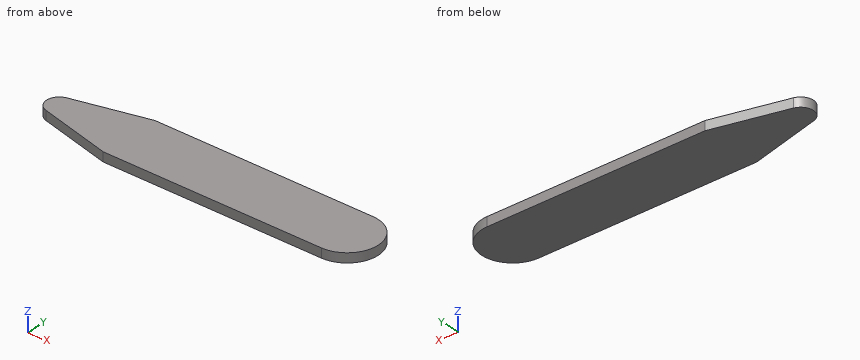
from build123d import *

# Parameters (mm, degrees)
F0_W     = 36
F0_H     = 10
F1_DEPTH = 1.5


with BuildPart() as f1:
    # F0 (on Top) → F1 (new body)
    with BuildSketch(Plane.XY):
        Rectangle(F0_W, F0_H)
        with BuildLine():
            Line((18, 5), (18, -5))
            ThreePointArc((18, -5), (23, 0), (18, 5))
        make_face()
        with BuildLine():
            Line((-30, -2), (-18, -5))
            Line((-18, -5), (-18, 5))
            Line((-18, 5), (-30, 2))
            ThreePointArc((-30, 2), (-31.561553, 0), (-30, -2))
        make_face()
    extrude(amount=F1_DEPTH)


solid = f1.part
CAD build for the part. Positions are in the model's coordinates, mm. Round coordinates to 2 decimals unless told otherwise and drop trailing zeros. Loops run counter-clockwise (first coordinate to the right, second up) from the corner with the lowest first, then second, coordinate; pieces in that order, holes last. Notation, with made-up numbers: (31, -32.5) - (81, -32.5) arc R9 ccw to (81, -18.5) - close; hole circle Ø7 at (16, 74.25). An arc over 180 degrees is marked (long way). Put each result on its own line as item: value.
1. Slice it at A-A on z = 0.8. List the corners of the cut face in (x, y), and give its area (3 significant figures).
Geometry check:
outline: (-30, -2) - (-18, -5) - (18, -5) arc R5 ccw to (18, 5) - (-18, 5) - (-30, 2) arc R2.06 ccw to start
area: 488 mm²
2. Wall check: line 1 (X direction, y = -1.75, z = 0.25); line 2 (Y direction, x = -26.5, z = 1.3) (3 decimals); line 3 (Y direction, x = -27.5, z = 1.35) (3 decimals). Give the ranges that are in metal, low to high.
Geometry check:
line 1: -30.59 to 22.68
line 2: -2.875 to 2.875
line 3: -2.625 to 2.625
3. Slice it at B-B on x = -23. List the corners of the cut face in (y, z).
Geometry check:
outline: (-3.75, 0) - (3.75, 0) - (3.75, 1.5) - (-3.75, 1.5) - close
4. Slice it at C-C on y = 3. List the corners of the cut face in (x, z), and give its area (3 significant figures).
Geometry check:
outline: (-26, 0) - (22, 0) - (22, 1.5) - (-26, 1.5) - close
area: 72.0 mm²
